Could you check a few things on this model? Use its own coordinates, in mm. A direction names the side the tool comes from. Coordinates: 2 decimals unless noted, no trailing zeros. Write each loop counter-clockwise with the first axis right and the second up, starting at its lowest first coordinate (ties: lowest second). Pieces come first, ordered by that corner, then holes.
Item 1: For P1, Ø8, axis at x = 42.5, y = 26, coming from the -Z side; P2, Ø5, axis at x = 10.5, y = 73.5, coming from the +Z side, each with a flat end and sliding along its axis, tell me the tip position at first contact or that it passes through.
Item 2: I want a section at A-A on x = 30. Please give me the cut outline in (y, z), then the cut area to 3 significant figures.
Item 3: I want a section at B-B on y = 55. Please give me the cut outline in (x, z).
Item 4: If I drill on probe 1 along Y at (x, z) = (25, 7.25); probe 2 along Z at (x, y) = (37, 8); probe 3 along Y at (x, z) = (30, 2.8), over which ranges is the centre line in solid material (lowest first)?
Item 5: I want a section at C-C on x = 50. Please give me the cut outline in (y, z), then the cut area to 3 significant figures.
Item 6: I want a section at D-D on y = 20. Please give me the cut outline in (x, z), then the cut area to 3 significant figures.
Item 7: Which directions (+Z, -Z, +X, -X, +Y, -Y) give clear straight access to the entire face, cutting with the end or side of a thin tool? Please do faces 1 (the flat face through (43.053, 39.685, 1.972)), 2 (the flat face through (30, 78, 9)), 3 (the flat face through (30, 0, 7)).
Item 8: Thinking about a two-plate mould opening in X: for faces 4 (the flat face through (30, 31, 15)), 5 (the flat face through (60, 54, 7)), 6 (the flat face through (40.942, 44.027, 1.972)), which applies, +X half, -X half, draft (parallel to the pull), parting line (faces both ways), or undercut?
from build123d import *

# Parameters (mm, degrees)
BOX_W                   = 46
BOX_H                   = 46
BOX_DEPTH               = 20
CYLINDER001_R           = 4.25
CYLINDER001_DEPTH       = 76
CYLINDER001_PITCH_ANGLE = 90
CYLINDER_R              = 4.25
CYLINDER_DEPTH          = 76
CYLINDER_PITCH_ANGLE    = 90
SKETCH_W                = 60
SKETCH_H                = 110
SKETCH_R                = 4.25
SKETCH_R_2              = 13
PAD_DEPTH               = 15


with BuildPart() as cubo:
    # Box → Box (new body)
    with BuildSketch(Plane(origin=(7.5, 32, 4), x_dir=(1, 0, 0), z_dir=(0, 0, 1))):
        with Locations((23, 23)):
            Rectangle(BOX_W, BOX_H)
    extrude(amount=BOX_DEPTH)


with BuildPart() as cilindro001:
    # Cylinder001 → Cylinder001 (new body)
    with BuildSketch(Plane.XY):
        Circle(CYLINDER001_R)
    extrude(amount=CYLINDER001_DEPTH)


with BuildPart() as cilindro001_1:
    # Cylinder001 pitch: moved
    add(cilindro001.part.rotate(Axis((0, 0, 0), (0, 1, 0)), CYLINDER001_PITCH_ANGLE))


with BuildPart() as cilindro001_2:
    # Cylinder001 placement: moved
    add(cilindro001_1.part.moved(Location((-1, 8, 7.5))))


with BuildPart() as cilindro:
    # Cylinder → Cylinder (new body)
    with BuildSketch(Plane.XY):
        Circle(CYLINDER_R)
    extrude(amount=CYLINDER_DEPTH)


with BuildPart() as cilindro_1:
    # Cylinder pitch: moved
    add(cilindro.part.rotate(Axis((0, 0, 0), (0, 1, 0)), CYLINDER_PITCH_ANGLE))


with BuildPart() as cilindro_2:
    # Cylinder placement: moved
    add(cilindro_1.part.moved(Location((-1, 102, 7.5))))


with BuildPart() as cut002:
    # Sketch → Pad (new body)
    with BuildSketch(Plane.XY):
        with Locations((30, 55)):
            Rectangle(SKETCH_W, SKETCH_H)
        with Locations((10, 20)):
            Circle(SKETCH_R, mode=Mode.SUBTRACT)
        with Locations((50, 20)):
            Circle(SKETCH_R, mode=Mode.SUBTRACT)
        with Locations((10, 90)):
            Circle(SKETCH_R, mode=Mode.SUBTRACT)
        with Locations((50, 90)):
            Circle(SKETCH_R, mode=Mode.SUBTRACT)
        with Locations((30, 55)):
            Circle(SKETCH_R_2, mode=Mode.SUBTRACT)
        Polygon((39.826039, 67.088781), (46.19, 73.452742), (48.452742, 71.19), (42.088781, 64.826039), align=None, mode=Mode.SUBTRACT)
        Polygon((39.826039, 42.911219), (42.088781, 45.173961), (48.452742, 38.81), (46.19, 36.547258), align=None, mode=Mode.SUBTRACT)
        Polygon((11.547258, 71.19), (13.81, 73.452742), (20.173961, 67.088781), (17.911219, 64.826039), align=None, mode=Mode.SUBTRACT)
        Polygon((11.547258, 38.81), (17.911219, 45.173961), (20.173961, 42.911219), (13.81, 36.547258), align=None, mode=Mode.SUBTRACT)
    extrude(amount=PAD_DEPTH)

    # Cut: cut Cilindro
    add(cilindro_2.part, mode=Mode.SUBTRACT)

    # Cut001: cut Cilindro001
    add(cilindro001_2.part, mode=Mode.SUBTRACT)

    # Cut002: cut Cubo
    add(cubo.part, mode=Mode.SUBTRACT)


solid = cut002.part
Response values:
1. P1: stops at z = 0
1. P2: stops at z = 4
2. outline: (0, 0) - (42, 0) - (42, 4) - (32, 4) - (32, 15) - (0, 15) - close; (68, 0) - (110, 0) - (110, 15) - (78, 15) - (78, 4) - (68, 4) - close; hole circle Ø8.5 at (8, 7.5); hole circle Ø8.5 at (102, 7.5)
2. area: 927 mm2
3. outline: (0, 0) - (17, 0) - (17, 4) - (7.5, 4) - (7.5, 15) - (0, 15) - close; (43, 0) - (60, 0) - (60, 15) - (53.5, 15) - (53.5, 4) - (43, 4) - close
4. probe 1: y = 0 to 3.76, 12.24 to 32, 78 to 97.76, 106.24 to 110
4. probe 2: z = 0 to 3.25, 11.75 to 15
4. probe 3: y = 0 to 42, 68 to 110
5. outline: (0, 0) - (15.75, 0) - (15.75, 15) - (0, 15) - close; (24.25, 0) - (85.75, 0) - (85.75, 15) - (78, 15) - (78, 4) - (32, 4) - (32, 15) - (24.25, 15) - close; (94.25, 0) - (110, 0) - (110, 15) - (94.25, 15) - close; hole circle Ø8.5 at (8, 7.5); hole circle Ø8.5 at (102, 7.5)
5. area: 776 mm2
6. outline: (0, 0) - (5.75, 0) - (5.75, 15) - (0, 15) - close; (14.25, 0) - (45.75, 0) - (45.75, 15) - (14.25, 15) - close; (54.25, 0) - (60, 0) - (60, 15) - (54.25, 15) - close
6. area: 645 mm2
7. face 1: +Z, -Z
7. face 2: +Z
7. face 3: +Z, -Z, +X, -X, -Y
8. face 4: draft
8. face 5: +X half
8. face 6: undercut
